Can you work these out from the model? Positions are in its coordinate system, mm. A direction names the side the tool comes from. Give positions to 0.01 mm unless a question says otherwise; leave off trailing zeros. Loops run counter-clockwise (first coordinate to the right, second up) from the corner with the lowest first, then second, coordinate; pieces in that order, holes last. Notation, with made-up numbers: (49.5, 14.25) - (67.5, 14.25) arc R21 cw to (67.5, 47.25) - close; hole circle Ø2 at (81.5, 6.25). An arc over 180 degrees is marked (long way). Write item = value, one per line.
from build123d import *

# Parameters (mm, degrees)
RESSALTO_EXTRUS_O1_DEPTH = 4
FILETE3_R                = 8
ESBO_O2_R                = 1.65
ESBO_O2_R_2              = 5
CORTE_EXTRUS_O1_DEPTH    = 40.102429592
FILETE12_SIZE            = 5
FILETE12_SIZE_2          = 12
FILETE14_R               = 2
ESBO_O3_W                = 9
ESBO_O3_H                = 13
CORTE_EXTRUS_O2_DEPTH    = 40.102429743
FILETE15_R               = 8
FILETE16_SIZE            = 3
FILETE16_SIZE_2          = 1.5


# Some blends are built 0.0001 mm under size
with BuildPart() as part:
    # Esboço1 → Ressalto-extrusão1 (new body)
    with BuildSketch(Plane.XY):
        Polygon((0, 0), (25, 0), (25, 28), (-27, 28), (-27, 13), (0, 13), align=None)
    extrude(amount=RESSALTO_EXTRUS_O1_DEPTH)

    # Filete3
    filete3_edges = [part.edges().sort_by_distance(p)[0] for p in [
        (0, 0, 2),
    ]]
    fillet(filete3_edges, radius=FILETE3_R)

    # Esboço2 → Corte-extrusão1 (cut, through all)
    with BuildSketch(Plane.XY.offset(4)):
        with Locations((-21.2, 21)):
            Circle(ESBO_O2_R)
        with Locations((8, 8)):
            Circle(ESBO_O2_R_2)
        with Locations((17.810708435, 20)):
            Circle(ESBO_O2_R_2)
    extrude(amount=-CORTE_EXTRUS_O1_DEPTH, mode=Mode.SUBTRACT)

    # Filete12
    # an asymmetric fillet: 12, 5 mm, written as the material it takes off along each edge
    with BuildSketch(Plane(origin=(-27, 28, -30), x_dir=(1, 0, 0), z_dir=(0, 0, 1))) as filete12_piece_1:
        with BuildLine():
            Bezier((FILETE12_SIZE, 0), (0, 0), (0, -FILETE12_SIZE_2), weights=[1, 0.707106781, 1])
            Line((0, -FILETE12_SIZE_2), (0, 0))
            Line((0, 0), (FILETE12_SIZE, 0))
        make_face()
    extrude(amount=64, mode=Mode.SUBTRACT)

    # Filete14
    filete14_edges = [part.edges().sort_by_distance(p)[0] for p in [
        (0, 13, 2),
    ]]
    fillet(filete14_edges, radius=FILETE14_R)

    # Esboço3 → Corte-extrusão2 (cut, through all)
    with BuildSketch(Plane.XY.offset(4)):
        with Locations((20.5, 6.5)):
            Rectangle(ESBO_O3_W, ESBO_O3_H)
    extrude(amount=-CORTE_EXTRUS_O2_DEPTH, mode=Mode.SUBTRACT)

    # Filete15
    filete15_edges = [part.edges().sort_by_distance(p)[0] for p in [
        (16, 0, 2),
    ]]
    fillet(filete15_edges, radius=FILETE15_R - 0.0001)  # a hair under: the kernel refuses the full size

    # Filete16
    # an asymmetric fillet: 3, 1.5 mm, written as the material it adds along each edge
    with BuildSketch(Plane(origin=(16, 13, 4), x_dir=(0, -1, 0), z_dir=(0, 0, -1))) as filete16_piece_1:
        with BuildLine():
            Bezier((FILETE16_SIZE, 0), (0, 0), (0, -FILETE16_SIZE_2), weights=[1, 0.707106781, 1])
            Line((0, -FILETE16_SIZE_2), (0, 0))
            Line((0, 0), (FILETE16_SIZE, 0))
        make_face()
    extrude(amount=4)


solid = part.part
Q1. Imagine slicing it at A-A, the plane x = 22. Write out the boundary of the cut face in (y, z), then the cut area to 3 significant figures.
Output:
outline = (13, 0) - (17.27, 0) - (17.27, 4) - (13, 4) - close; (22.73, 0) - (28, 0) - (28, 4) - (22.73, 4) - close
area = 38.2 mm2
Q2. I need wall thicknesses on L1, parallel to Y at x = 8, z = 1.2; L2, parallel to Y at x = -14.5, z = 1.7; L3, parallel to X at y = 5, z = 1.2. Which ranges of each line are inside material? Lowest first, please.
Output:
L1 = 0 to 3, 13 to 28
L2 = 13 to 28
L3 = 0.58 to 4, 12 to 15.42
Q3. Which directions (+Z, -Z, +X, -X, +Y, -Y) give clear straight access to the entire face, cutting with the end or side of a thin tool? Please do faces 4 (the flat face through (0, 10, 2)), 5 (the cylindrical face through (12.77, 9.5, 2.03)), 6 (the flat face through (21, 13, 2)).
Output:
face_4 = +Z, -Z, -X, -Y
face_5 = +Z, -Z
face_6 = +Z, -Z, +X, -Y
Q4. Imagine slicing it at C-C, the plane x = -6.5. Write out the boundary of the cut face in (y, z), then the cut area to 3 significant figures.
Output:
outline = (13, 0) - (28, 0) - (28, 4) - (13, 4) - close
area = 60.0 mm2
Q5. For pin 1 (2 mm diameter, centred on x = 21.5, z = 1.5, fed in from -Y); pin 2 (2 mm diameter, centred on y = 9.5, z = 3, fed in from +X); pin 3 (1.5 mm diameter, centred on y = 9, z = 1.5, fed in from -X), each with a flat end and sliding along its axis, tell me the tip position at first contact or that it passes through.
Output:
pin_1 = 13
pin_2 = 16.02
pin_3 = 0
Q6. We'd pull the mould along X, two halves only. Please class faces 1 (the cylindrical face through (13.84, 16.96, 2.03)), 2 (the cylindrical face through (2.406, 2.281, 2.028)), 3 (the flat face through (2, 28, 2)): released by +X, released by -X, zero draft, split by the parting line, or undercut.
Output:
face_1 = undercut
face_2 = released by -X
face_3 = zero draft
Q7. Imagine slicing it at B-B, the plane z = 1.5. Give the number of separate pieces and of enclosed holes in the cut face, then the cut area to 3 significant figures.
Output:
separate_pieces = 1
enclosed_holes = 3
area = 784 mm2
